Part print with two shaded views. Sizes in mm from the minimum x, y, z corner. A direction names the side the tool comes from. Give positions to 0.01 mm unless a question says otherwise; leave off trailing zeros. Loops run counter-clockwise (first coordinate to the right, second up) from the corner with the lowest first, then second, coordinate; pieces in that order, holes last. Notation, with made-up numbers: M -14.5,35.25 L 29.5,35.25 A8 cw 29.5,45.25 Z; hole C 0.5,6.25 d10. An arc over 180 degrees is marked long. Answer as a JSON object with one key per item and string values. Group by question number.
1. 3-axis set-ups, long thin cutter, end or side, ignore diameter. For the marked faces 1, 2 and 3: which of +Z, -Z, +X, -X, +Y, -Y reach the whole face in a straight line?
2. Slice it at B-B (x = 7.75). List the corners of the cut face in (y, z), then the cut area to 3 significant figures.
3. Slice it at D-D (y = 3.25). List the corners of the cut face in (x, z).
4. Mould opens along X. For the marked faces 4, 5 and 6 say: released by +X, released by -X, zero draft, split by the parting line, or undercut.
5. Drop flat-ended pins along their axis: pin 1 Ø1.5 at (x, z) = (1.5, 6.5) entering from -Y; pin 2 Ø1 at (y, z) = (3, 5) entering from -X. Give the stop position or say it passes through.
6. Drill centre lines: line 1 along Y through (x, z) = (9.25, 5.25); line 2 along X through (y, z) = (3.5, 1.75); line 3 along Y through (x, z) = (13, 9.75). Where is each one in solid material? Low to high. Write a range as [from, to].
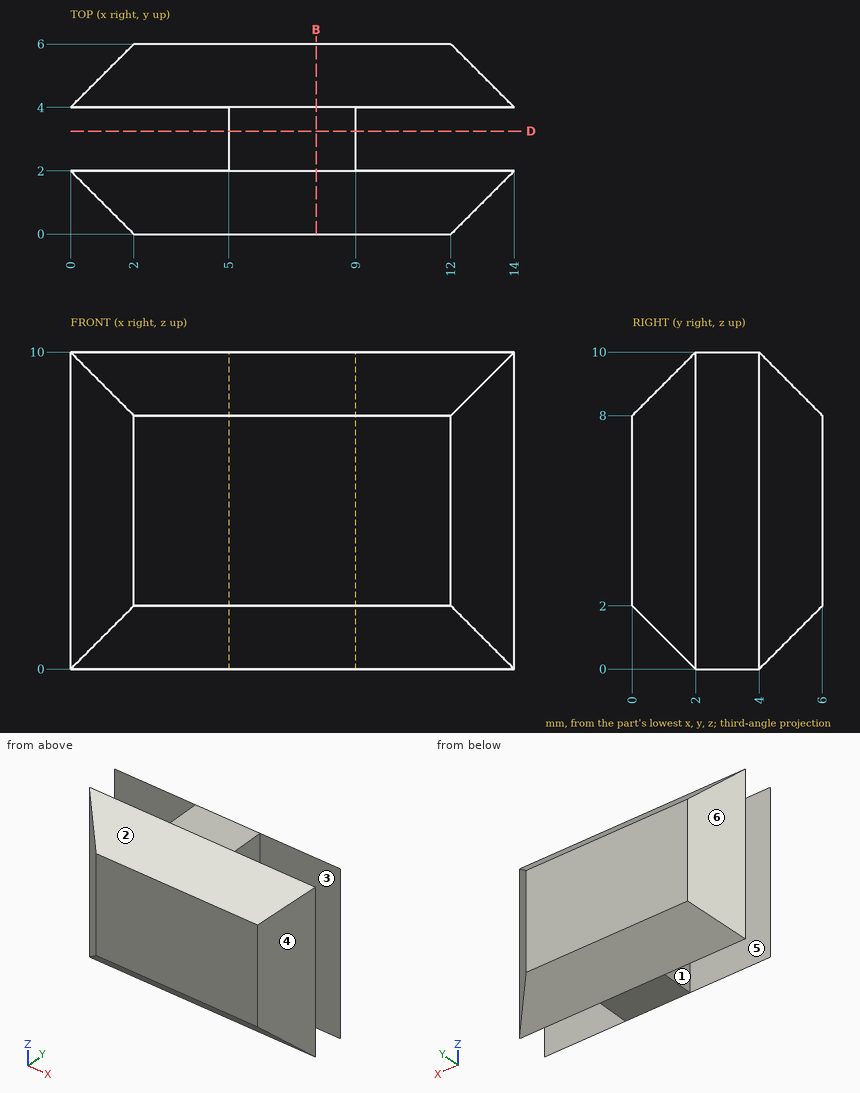
Established:
{
 "1": {"face 1": "+Z, -Z, -X", "face 2": "+Z, +X, -X, -Y", "face 3": "+Z, -Z, +X"},
 "2": {"outline": "M 0,2 L 2,0 L 4,0 L 6,2 L 6,8 L 4,10 L 2,10 L 0,8 Z", "area": "52.0 mm^2"},
 "3": {"outline": "M 5,0 L 9,0 L 9,10 L 5,10 Z"},
 "4": {"face 4": "released by +X", "face 5": "zero draft", "face 6": "released by -X"},
 "5": {"pin 1": "stops at y = 0", "pin 2": "stops at x = 5"},
 "6": {"line 1": "y = [0, 2], [4, 6]", "line 2": "x = [5, 9]", "line 3": "y = [1.75, 2], [4, 4.25]"}
}
